```python
from build123d import *

# Parameters (mm, degrees)
SKETCH_1_R           = 3
SKETCH_1_W           = 90
SKETCH_1_H           = 120
SKETCH_1_R_2         = 10
SKETCH_1_R_3         = 7.5
EXTRUDE_2_DEPTH      = 3
EXTRUDE_START        = -10
SKETCH_2_R           = 7.5
EXTRUDE_3_DEPTH      = 10
CUT_EXTRUDE_1_DEPTH  = 10
EXTRUDE_START_2      = -3
SKETCH_4_R           = 10
EXTRUDE_4_DEPTH      = 3
SKETCH_6_W           = 7
SKETCH_6_H           = 14.142135624
CUT_EXTRUDE_5_DEPTH  = 333.489097566
SKETCH_7_W           = 90
SKETCH_7_H           = 120
EXTRUDE_5_DEPTH      = 3
SKETCH_8_W           = 10
SKETCH_8_H           = 50
EXTRUDE_6_DEPTH      = 30
SKETCH_9_R           = 8
CUT_EXTRUDE_6_DEPTH  = 30
SKETCH_10_R          = 3
EXTRUDE_7_DEPTH      = 3
SKETCH_11_R          = 3
CUT_EXTRUDE_7_DEPTH  = 3
SKETCH_12_R          = 3
EXTRUDE_8_DEPTH      = 3
SKETCH_13_R          = 3
CUT_EXTRUDE_8_DEPTH  = 3
SKETCH_14_R          = 3
CUT_EXTRUDE_9_DEPTH  = 10
SKETCH_15_R          = 3
CUT_EXTRUDE_10_DEPTH = 231.922064775
SKETCH_16_R          = 3
EXTRUDE_10_DEPTH     = 3
SKETCH_17_R          = 3
CUT_EXTRUDE_11_DEPTH = 231.922064775
SKETCH_18_R          = 5
CUT_EXTRUDE_12_DEPTH = 10
SKETCH_19_W          = 30
SKETCH_19_H          = 50
CUT_EXTRUDE_13_DEPTH = 10
EXTRUDE_11_DEPTH     = 3
EXTRUDE_12_DEPTH     = 3
CUT_EXTRUDE_14_DEPTH = 3
SKETCH_23_W          = 90
SKETCH_23_H          = 120
CUT_EXTRUDE_15_DEPTH = 3
SKETCH_24_R          = 10
SKETCH_24_R_2        = 7.5
CUT_EXTRUDE_16_DEPTH = 3
SKETCH_25_R          = 1.5
CUT_EXTRUDE_17_DEPTH = 10
SKETCH_26_R          = 4
CUT_EXTRUDE_18_DEPTH = 10
SKETCH_27_R          = 4
CUT_EXTRUDE_19_DEPTH = 10


with BuildPart() as part:
    # 草图1 → 凸台-拉伸2 (new body)
    # profile 1 of 9: a face of its own
    with BuildSketch(Plane.XY):
        Polygon((195, -115), (195, 115), (190, 115), (190, 120), (115, 120), (115, 75), (75, 75), (-90, 75), (-130, 75), (-130, 120), (-175, 120), (-175, 90), (-195, 90), (-195, -90), (-175, -90), (-175, -120), (-130, -120), (-130, -75), (-90, -75), (75, -75), (115, -75), (115, -120), (190, -120), (190, -115), align=None)
        with Locations((-184.089468205, -70)):
            Circle(SKETCH_1_R, mode=Mode.SUBTRACT)
        with Locations((-87, -69)):
            Circle(SKETCH_1_R, mode=Mode.SUBTRACT)
        with Locations((-184.089468205, 70)):
            Circle(SKETCH_1_R, mode=Mode.SUBTRACT)
        with Locations((-87, 69)):
            Circle(SKETCH_1_R, mode=Mode.SUBTRACT)
        Rectangle(SKETCH_1_W, SKETCH_1_H, mode=Mode.SUBTRACT)
        with Locations((75, 0)):
            Circle(SKETCH_1_R_2, mode=Mode.SUBTRACT)
        with Locations((117.5, 0)):
            Circle(SKETCH_1_R_3, mode=Mode.SUBTRACT)
    # profile 2 of 9: a face of its own
    with BuildSketch(Plane.XY):
        Polygon((-130, 120), (-90, 75), (-130, 75), align=None)
    # profile 3 of 9: a face of its own
    with BuildSketch(Plane.XY):
        Polygon((-175, 120), (-175, 90), (-195, 90), align=None)
    # profile 4 of 9: a face of its own
    with BuildSketch(Plane.XY):
        Polygon((-175, -120), (-195, -90), (-175, -90), align=None)
    # profile 5 of 9: a face of its own
    with BuildSketch(Plane.XY):
        Polygon((-130, -120), (-130, -75), (-90, -75), align=None)
    # profile 6 of 9: a face of its own
    with BuildSketch(Plane.XY):
        Polygon((115, -120), (75, -75), (115, -75), align=None)
        with Locations((104.379549532, -93)):
            Circle(SKETCH_1_R, mode=Mode.SUBTRACT)
    # profile 7 of 9: a face of its own
    with BuildSketch(Plane.XY):
        Polygon((115, 120), (115, 75), (75, 75), align=None)
        with Locations((104.379549532, 93)):
            Circle(SKETCH_1_R, mode=Mode.SUBTRACT)
    # profile 8 of 9: a face of its own
    with BuildSketch(Plane.XY):
        Polygon((190, 120), (195, 115), (190, 115), align=None)
    # profile 9 of 9: a face of its own
    with BuildSketch(Plane.XY):
        Polygon((190, -115), (190, -120), (195, -115), align=None)
    extrude(amount=EXTRUDE_2_DEPTH)

    # 草图2 → 凸台-拉伸3 (add)
    with BuildSketch(Plane.XY.offset(3).offset(EXTRUDE_START)):
        with Locations((117.5, 0)):
            Circle(SKETCH_2_R)
    extrude(amount=EXTRUDE_3_DEPTH)

    # 草图3 → 切除-拉伸1 (cut)
    with BuildSketch(Plane.XY.offset(3)):
        Polygon((115, 120), (115, -120), (190, -120), (195, -115), (195, 115), (190, 120), align=None)
        Polygon((115, -120), (115, -114.375), (110, -114.375), align=None)
        Polygon((115, 114.376866735), (115, 120), (110.00165932, 114.376866735), align=None)
    extrude(amount=-CUT_EXTRUDE_1_DEPTH, mode=Mode.SUBTRACT)

    # 草图4 → 凸台-拉伸4 (add)
    with BuildSketch(Plane.XY.offset(3).offset(EXTRUDE_START_2)):
        with Locations((75, 0)):
            Circle(SKETCH_4_R)
    extrude(amount=EXTRUDE_4_DEPTH)

    # 草图6 → 切除-拉伸5 (cut, through all)
    with BuildSketch(Plane(origin=(115, 0, 0), x_dir=(0, 0, -1), z_dir=(1, 0, 0))):
        with Locations((3.5, 0)):
            Rectangle(SKETCH_6_W, SKETCH_6_H)
    extrude(amount=-CUT_EXTRUDE_5_DEPTH, mode=Mode.SUBTRACT)

    # 草图7 → 凸台-拉伸5 (add)
    with BuildSketch(Plane.XY.offset(3)):
        Rectangle(SKETCH_7_W, SKETCH_7_H)
    extrude(amount=-EXTRUDE_5_DEPTH)

    # 草图8 → 凸台-拉伸6 (add)
    with BuildSketch(Plane.XY.offset(3)):
        with Locations((110, 0)):
            Rectangle(SKETCH_8_W, SKETCH_8_H)
    extrude(amount=EXTRUDE_6_DEPTH)

    # 草图9 → 切除-拉伸6 (cut)
    with BuildSketch(Plane(origin=(115, 0, 0), x_dir=(0, 0, -1), z_dir=(1, 0, 0))):
        with Locations((-17.93158575, 0)):
            Circle(SKETCH_9_R)
    extrude(amount=-CUT_EXTRUDE_6_DEPTH, mode=Mode.SUBTRACT)

    # 草图10 → 凸台-拉伸7 (add)
    with BuildSketch(Plane.XY.offset(3).offset(EXTRUDE_START_2)):
        with Locations((104.379549532, -93)):
            Circle(SKETCH_10_R)
        with Locations((104.379549532, 93)):
            Circle(SKETCH_10_R)
    extrude(amount=EXTRUDE_7_DEPTH)

    # 草图11 → 切除-拉伸7 (cut)
    with BuildSketch(Plane.XY.offset(3)):
        with Locations((100, -88.073006777)):
            Circle(SKETCH_11_R)
        with Locations(Location((100, 88.073006777, 0), (0, 0, 180))):
            Circle(SKETCH_11_R)
    extrude(amount=-CUT_EXTRUDE_7_DEPTH, mode=Mode.SUBTRACT)

    # 草图12 → 凸台-拉伸8 (add)
    with BuildSketch(Plane.XY.offset(3).offset(EXTRUDE_START_2)):
        with Locations((-87, 69)):
            Circle(SKETCH_12_R)
        with Locations((-87, -69)):
            Circle(SKETCH_12_R)
    extrude(amount=EXTRUDE_8_DEPTH)

    # 草图13 → 切除-拉伸8 (cut)
    with BuildSketch(Plane.XY.offset(3)):
        with Locations((-90, 65)):
            Circle(SKETCH_13_R)
        with Locations(Location((-90, -65, 0), (0, 0, 180))):
            Circle(SKETCH_13_R)
    extrude(amount=-CUT_EXTRUDE_8_DEPTH, mode=Mode.SUBTRACT)

    # 草图14 → 切除-拉伸9 (cut)
    with BuildSketch(Plane.XY.offset(3)):
        with BuildLine():
            ThreePointArc((-159.5, 88), (-160.378679656, 90.121320344), (-162.5, 91))
            Line((-162.5, 91), (-162.5, 85))
            ThreePointArc((-162.5, 85), (-160.378679656, 85.878679656), (-159.5, 88))
        make_face()
        with BuildLine():
            Line((-162.5, 85), (-162.5, 91))
            ThreePointArc((-162.5, 91), (-165.5, 88), (-162.5, 85))
        make_face()
        with Locations((-162.5, -88)):
            Circle(SKETCH_14_R)
    extrude(amount=-CUT_EXTRUDE_9_DEPTH, mode=Mode.SUBTRACT)

    # 草图15 → 切除-拉伸10 (cut, through all)
    with BuildSketch(Plane.XY.offset(3)):
        with Locations((-162.5, -93)):
            Circle(SKETCH_15_R)
        with Locations((-162.5, -88)):
            Circle(SKETCH_15_R)
        with Locations((-162.5, 93)):
            Circle(SKETCH_15_R)
        with Locations((-162.5, 88)):
            Circle(SKETCH_15_R)
    extrude(amount=-CUT_EXTRUDE_10_DEPTH, mode=Mode.SUBTRACT)

    # 草图16 → 凸台-拉伸10 (add)
    with BuildSketch(Plane.XY.offset(3)):
        with Locations((-162.5, 88)):
            Circle(SKETCH_16_R)
        with Locations((-162.5, -88)):
            Circle(SKETCH_16_R)
    extrude(amount=-EXTRUDE_10_DEPTH)

    # 草图17 → 切除-拉伸11 (cut, through all)
    with BuildSketch(Plane.XY.offset(3)):
        with Locations((-162.5, 93)):
            Circle(SKETCH_17_R)
        with Locations((-162.5, -93)):
            Circle(SKETCH_17_R)
    extrude(amount=-CUT_EXTRUDE_11_DEPTH, mode=Mode.SUBTRACT)

    # 草图18 → 切除-拉伸12 (cut)
    with BuildSketch(Plane.XY.offset(3)):
        with Locations((-170, 22.5)):
            Circle(SKETCH_18_R)
        with Locations((-170, -22.5)):
            Circle(SKETCH_18_R)
    extrude(amount=-CUT_EXTRUDE_12_DEPTH, mode=Mode.SUBTRACT)

    # 草图19 → 切除-拉伸13 (cut)
    with BuildSketch(Plane.ZY.offset(-105)):
        with Locations((18, 0)):
            Rectangle(SKETCH_19_W, SKETCH_19_H)
    extrude(amount=-CUT_EXTRUDE_13_DEPTH, mode=Mode.SUBTRACT)

    # 草图20 → 凸台-拉伸11 (add)
    with BuildSketch(Plane.XY.offset(3)):
        Polygon((195, 0.000933368), (115, 0.000933368), (115, -114.375), (115, -119.998133265), (195, -119.998133265), align=None)
        Polygon((115, 120), (115, 114.376866735), (115, 0.000933368), (195, 0.000933368), (195, 120), align=None)
    extrude(amount=-EXTRUDE_11_DEPTH)

    # 草图21 → 凸台-拉伸12 (add)
    with BuildSketch(Plane.XY.offset(3)):
        Polygon((115, 120), (110.00165932, 114.376866735), (115, 114.376866735), align=None)
        Polygon((110, -114.375), (115, -119.998133265), (115, -114.375), align=None)
    extrude(amount=-EXTRUDE_12_DEPTH)

    # 草图22 → 切除-拉伸14 (cut)
    with BuildSketch(Plane.XY.offset(3)):
        Polygon((195, 115), (195, 120), (190, 120), align=None)
        Polygon((195, -120), (190, -120), (195, -115), align=None)
    extrude(amount=-CUT_EXTRUDE_14_DEPTH, mode=Mode.SUBTRACT)

    # 草图23 → 切除-拉伸15 (cut)
    with BuildSketch(Plane.XY.offset(3)):
        Rectangle(SKETCH_23_W, SKETCH_23_H)
    extrude(amount=-CUT_EXTRUDE_15_DEPTH, mode=Mode.SUBTRACT)

    # 草图24 → 切除-拉伸16 (cut)
    with BuildSketch(Plane.XY.offset(3)):
        with Locations((75, 0)):
            Circle(SKETCH_24_R)
        with Locations((117.5, 0)):
            Circle(SKETCH_24_R_2)
    extrude(amount=-CUT_EXTRUDE_16_DEPTH, mode=Mode.SUBTRACT)

    # 草图25 → 切除-拉伸17 (cut)
    with BuildSketch(Plane.XY.offset(3)):
        with Locations((-72.75, 0)):
            Circle(SKETCH_25_R)
    extrude(amount=-CUT_EXTRUDE_17_DEPTH, mode=Mode.SUBTRACT)

    # 草图26 → 切除-拉伸18 (cut)
    with BuildSketch(Plane.XY.offset(3)):
        with Locations((-170, 0)):
            Circle(SKETCH_26_R)
    extrude(amount=-CUT_EXTRUDE_18_DEPTH, mode=Mode.SUBTRACT)

    # 草图27 → 切除-拉伸19 (cut)
    with BuildSketch(Plane.XY.offset(3)):
        with Locations((0, -67.5)):
            Circle(SKETCH_27_R)
        with Locations((0, 67.5)):
            Circle(SKETCH_27_R)
        with Locations((-170, 0)):
            Circle(SKETCH_27_R)
        with Locations((170, 0)):
            Circle(SKETCH_27_R)
    extrude(amount=-CUT_EXTRUDE_19_DEPTH, mode=Mode.SUBTRACT)


solid = part.part
```
Here's how the part is built. I have some questions about the finished solid (model axes, mm). A direction names the side the tool comes from. Round coordinates to 2 decimals unless told otherwise and drop trailing zeros. Order: outer loops, then holes, each group sorted by start corner. A loop starts at its lowest first (then second) coordinate and runs counter-clockwise, first axis right, second up. Notation, with made-up numbers: (66.5, 71.5) -> (76.5, 71.5) arc R16 ccw to (76.5, 81.5) -> close; hole circle Ø5 at (1.25, 46). An arc over 180 degrees is marked (long way). Use a Markdown table: item, result. Add a question column.
(1) Suppose I cut it at C-C, the plane z = 2.1. Count the separate pieces of the cut face and the enclosed holes in it, and give its area (3 significant figures).
(2) I need wall thicknesses on line 1 along Y through (x, z) = (-90, 1.65); line 2 along X through (y, z) = (-89.5, 2.5); line 3 along X through (y, z) = (-39.5, 0.95). Which ranges of each line are inside material? Lowest first, please.
(3) For faces 4 (the face through (-109.72, -97.185, 1.479)), 5 (the face through (95.28, 97.815, 1.521)), 6 (the face through (-174, 19.5, 1.5)), which set-ups out of +Z, -Z, +X, -X, +Y, -Y let a thin tool reach every point of the face, with its end or its side?
(4) Suppose I cut it at B-B, the plane y = 52. Please give me the cut outline in (x, z), and give its area (3 significant figures).
(5) Suppose I cut it at A-A, the plane x = 170. Please give me the cut outline in (y, z).
(6) For pin 1 Ø7 at (x, y) = (0, 67.5) entering from +Z; pin 2 Ø5 at (x, y) = (-72.75, 0) entering from +Z; pin 3 Ø0.9 at (x, z) = (-18, 2) entering from +Y, each with a flat end and sliding along its axis, tell me the tip position at first contact or that it passes through.
(7) If we mould it in two halves opening along X, with no side actions, what happens to faces 1 (the face through (-46, 2, 0)), 2 (the face through (-0.867, -71.405, 1.521)), 3 (the face through (-185, 105, 1))? For each: released by +X, released by -X, zero draft, split by the parting line, or undercut.
Verdict:
| question | item | result |
|---|---|---|
| 1 | separate pieces | 1 |
| 1 | enclosed holes | 18 |
| 1 | area | 62,600 mm2 |
| 2 | line 1 | -75 to -68, -62 to 62, 68 to 75 |
| 2 | line 2 | -195 to -102.89, 87.89 to 97.36, 102.64 to 195 |
| 2 | line 3 | -195 to -45, 45 to 195 |
| 3 | face 4 | +Z, -Z, -Y |
| 3 | face 5 | +Z, -Z, +Y |
| 3 | face 6 | +Z, -Z |
| 4 | outline | (-195, 0) -> (-45, 0) -> (-45, 3) -> (-195, 3) -> close; (45, 0) -> (195, 0) -> (195, 3) -> (45, 3) -> close |
| 4 | area | 900 mm2 |
| 5 | outline | (-120, 0) -> (-4, 0) -> (-4, 3) -> (-120, 3) -> close; (4, 0) -> (120, 0) -> (120, 3) -> (4, 3) -> close |
| 6 | pin 1 | through |
| 6 | pin 2 | z = 3 |
| 6 | pin 3 | y = 75 |
| 7 | face 1 | zero draft |
| 7 | face 2 | undercut |
| 7 | face 3 | released by -X |
